Verification items for the finished model (mm, model axes). A direction names the side the tool comes from. Give positions to 0.01 mm unless a question says otherwise; leave off trailing zeros. Loops run counter-clockwise (first coordinate to the right, second up) from the corner with the lowest first, then second, coordinate; pieces in that order, holes last. Notation, with made-up numbers: M -1,1 L 13,1 A18 ccw 13,21 Z; hole C 40.25,-20.75 d1. An arc over 180 degrees is marked long. Write each question's results on one line, items separated by ' | '. Start each with the question number.
```python
from build123d import *

# Parameters (mm, degrees)
ESQUISSE1_W             = 15
ESQUISSE1_H             = 15
EXTRUSION1_DEPTH        = 100
ESQUISSE2_W             = 12
ESQUISSE2_H             = 12
EXTRUSION2_DEPTH        = 101.560926806
ESQUISSE3_R             = 1.5
ENL_V_MAT_EXTRU_1_DEPTH = 102.396498953
ESQUISSE4_R             = 1.5
ENL_V_MAT_EXTRU_2_DEPTH = 102.396498953
ESQUISSE5_R             = 1.5
ENL_V_MAT_EXTRU_3_DEPTH = 102.396498953


with BuildPart() as part:
    # Esquisse1 → Extrusion1 (new body)
    with BuildSketch(Plane.XY):
        Rectangle(ESQUISSE1_W, ESQUISSE1_H)
    extrude(amount=EXTRUSION1_DEPTH)

    # Esquisse2 → Extrusion2 (cut, through all)
    with BuildSketch(Plane.XY.offset(100)):
        Rectangle(ESQUISSE2_W, ESQUISSE2_H)
    extrude(amount=-EXTRUSION2_DEPTH, mode=Mode.SUBTRACT)

    # Esquisse3 → Enlèv. mat.-Extru.1 (cut, through all)
    with BuildSketch(Plane(origin=(7.5, 0, 0), x_dir=(0, 0, -1), z_dir=(1, 0, 0))):
        with Locations((-5, 0)):
            Circle(ESQUISSE3_R)
    extrude(amount=-ENL_V_MAT_EXTRU_1_DEPTH, mode=Mode.SUBTRACT)

    # Esquisse4 → Enlèv. mat.-Extru.2 (cut, through all)
    with BuildSketch(Plane(origin=(7.5, 0, 0), x_dir=(0, 0, -1), z_dir=(1, 0, 0))):
        with Locations((-20, 0)):
            Circle(ESQUISSE4_R)
    extrude(amount=-ENL_V_MAT_EXTRU_2_DEPTH, mode=Mode.SUBTRACT)

    # Esquisse5 → Enlèv. mat.-Extru.3 (cut, through all)
    with BuildSketch(Plane(origin=(7.5, 0, 0), x_dir=(0, 0, -1), z_dir=(1, 0, 0))):
        with Locations((-95, 0)):
            Circle(ESQUISSE5_R)
        with Locations((-80, 0)):
            Circle(ESQUISSE5_R)
    extrude(amount=-ENL_V_MAT_EXTRU_3_DEPTH, mode=Mode.SUBTRACT)


solid = part.part
```
1. Section check B-B, the plane y = -3.75. Record the boundary of the cut face in (x, z), plus the area to 3 significant figures.
2. Thickness scan on probe 1 along X at (y, z) = (4.75, 48); probe 2 along Y at (x, z) = (7.05, 95). Record the ranges inside material, lowest first.
3. Set-up check for faces 4 (the face through (6.76, 0.45, 93.57)), 5 (the face through (0, -6, 51)): record each of +Z, -Z, +X, -X, +Y, -Y from which the full face is reachable in a straight line by a thin tool's end or side.
4. Section check A-A, the plane z = 31. Record the boundary of the cut face in (x, y), plus the area to 3 significant figures.
5. Depth check by flat-ended pin: pin 1 Ø1.8 at (y, z) = (0, 95) entering from -X; pin 2 Ø2 at (x, y) = (1, -6) entering from -Z. Enter the tip coordinate at first touch or a pass-through.
6. Release check for a two-part mould opening along Y. For faces 1 (the face through (0, 7.5, 49)), 2 (the face through (0, -7.5, 49)), 3 (the face through (6.76, 0.45, 78.57)) record: released by +Y, released by -Y, zero draft, split by the parting line, or undercut.
7. Section check D-D, the plane z = 80. Record the boundary of the cut face in (x, y), plus the area to 3 significant figures.
Filled sheet:
1) outline: M -7.5,0 L -6,0 L -6,100 L -7.5,100 Z; M 6,0 L 7.5,0 L 7.5,100 L 6,100 Z | area: 300 mm2
2) probe 1: -7.5 to -6, 6 to 7.5 | probe 2: -7.5 to -1.5, 1.5 to 7.5
3) face 4: +X, -X | face 5: +Z, -Z
4) outline: M -7.5,-7.5 L 7.5,-7.5 L 7.5,7.5 L -7.5,7.5 Z; hole M -6,-6 L 6,-6 L 6,6 L -6,6 Z | area: 81.0 mm2
5) pin 1: through | pin 2: z = 0
6) face 1: released by +Y | face 2: released by -Y | face 3: undercut
7) outline: M -7.5,-7.5 L 7.5,-7.5 L 7.5,-1.5 L 6,-1.5 L 6,-6 L -6,-6 L -6,-1.5 L -7.5,-1.5 Z; M -7.5,1.5 L -6,1.5 L -6,6 L 6,6 L 6,1.5 L 7.5,1.5 L 7.5,7.5 L -7.5,7.5 Z | area: 72.0 mm2
